Read the model definition and answer for the solid it produces. Units are mm, in the model's axes. A direction names the side the tool comes from. Coordinates: 2 decimals unless noted, no trailing zeros. Loops run counter-clockwise (first coordinate to the right, second up) from the corner with the lowest first, then second, coordinate; pieces in that order, holes last. Notation, with made-up numbers: M 36.25,-24.5 L 79.25,-24.5 A22 ccw 79.25,8.5 Z; hole C 40,44.5 d7. An arc over 180 degrees is marked long. One line per item, written item: value. Start each with the question number.
Autodesk Inventor part; units mm, degrees
ref_plane "YZ Plane" through (0, 0, 0) normal (1, 0, 0) x (0, 1, 0)
ref_plane "XY Plane" through (0, 0, 0) normal (0, 0, 1) x (1, 0, 0)
sketch "Sketch1" plane through (0, 0, 0) normal (0, 1, 0) x (-1, 0, 0)
  line L0 (0, -144.8636) -> (0, 84.5516) construction
  line L1 (624.86, 0) -> (-675.46, 0) construction
  line L2 (338.2, 51.778) -> (439.1, -35.05)
  line L3 (439.1, -35.05) -> (421.2, -60.89)
  line L4 (421.2, -60.89) -> (242.5, -95.89)
  line L5 (242.5, -95.89) -> (-209.7, -95.89)
  line L6 (-209.7, -95.89) -> (-256.7, -112.09)
  line L7 (-256.7, -112.09) -> (-489.7, -112.09)
  line L8 (-489.7, -112.09) -> (-489.7, -49.69)
  line L9 (-489.7, -49.69) -> (-453.7, -40.3)
  line L10 (-453.7, -40.3) -> (-431.7, 3.13)
  line L11 (-431.7, 3.13) -> (-349.7, 51.778)
  line L12 (-349.7, 51.778) -> (338.2, 51.778)
  point P0 (0, 0)
  dimension "d0" = 51.778
  dimension "d1" = 35.05
  dimension "d2" = 60.89
  dimension "d3" = 95.89
  dimension "d4" = 95.89
  dimension "d5" = 112.09
  dimension "d6" = 112.09
  dimension "d8" = 40.3
  dimension "d9" = 49.69
  dimension "d10" = 3.13
  dimension "d11" = 51.778
  dimension "d12" = 338.2
  dimension "d13" = 439.1
  dimension "d14" = 421.2
  dimension "d15" = 242.5
  dimension "d16" = 489.7
  dimension "d17" = 256.7
  dimension "d18" = 209.7
  dimension "d19" = 489.7
  dimension "d20" = 453.7
  dimension "d21" = 431.7
  dimension "d22" = 349.7
extrude "Extrusion1" add sketch "Sketch1" along normal mid plane 52
properties part number "Friend_track_collision"
1) Section B-B (x = -142) is taken. Determine the outline of the cut face in (y, z), then the cut area to 3 significant figures.
2) Consider line 1 along Z through (x, y) = (28, 19.5); line 2 along X through (y, z) = (9.5, 20); line 3 along X through (y, z) = (5, -28). Determine where each line is inside the solid, lowest interval first.
3) Section A-A (y = -3) is taken. Determine the outline of the cut face in (x, z), then the cut area to 3 significant figures.
4) Section C-C (z = -9.5) is taken. Determine the outline of the cut face in (x, y), then the cut area to 3 significant figures.
5) A tool of negligible diameter and unlimited length cuts with its end or side. For faces 1 (the face through (32, 26, -29)), 2 (the face through (-20, 0, -95.89)), from which of +Z, -Z, +X, -X, +Y, -Y can it reach the whole face along a straight path? Write none if from no direction.
6) Flat-ended cylindrical pins translate along their axes: pin 1 (12 mm diameter, centred on y = 12, z = 8, fed in from +X); pin 2 (1.5 mm diameter, centred on y = 16.5, z = -12, fed in from -X); pin 3 (4 mm diameter, centred on x = 53, y = -2.5, fed in from -Z). Find the tip coordinate at first contact, or state that the pin passes through.
Results found:
1. outline: M -26,-95.89 L 26,-95.89 L 26,51.78 L -26,51.78 Z
1. area: 7,680 mm²
2. line 1: z = -95.89 to 51.78
2. line 2: x = -375.13 to 403.26
2. line 3: x = -430.91 to 447.47
3. outline: M -439.1,-35.05 L -421.2,-60.89 L -242.5,-95.89 L 209.7,-95.89 L 256.7,-112.09 L 489.7,-112.09 L 489.7,-49.69 L 453.7,-40.3 L 431.7,3.13 L 349.7,51.78 L -338.2,51.78 Z
3. area: 126,000 mm²
4. outline: M -409.41,-26 L 438.1,-26 L 438.1,26 L -409.41,26 Z
4. area: 44,100 mm²
5. face 1: +Z, -Z, +X, -X, +Y
5. face 2: -Z, -X, +Y, -Y
6. pin 1: stops at x = 432.27
6. pin 2: stops at x = -413.19
6. pin 3: stops at z = -95.89
